from build123d import *

# Parameters (mm, degrees)
ESBO_O1_R                     = 1.5
RESSALTO_EXTRUS_O1_DEPTH      = 9
RESSALTO_EXTRUS_O2_DEPTH      = 5
RESSALTO_EXTRUS_O2_DEPTH_BACK = 11
ESBO_O2_W                     = 11
ESBO_O2_H                     = 8
FILETE1_R                     = 2.5
CHANFRO1_SIZE                 = 2


with BuildPart() as part:
    # Esboço1 → Ressalto-extrusão1 (new body)
    with BuildSketch(Plane.XY):
        Polygon((-3, -3), (3, -3), (3, 3), (-3, 3), (-10, 3), (-10, -3), align=None)
        Circle(ESBO_O1_R, mode=Mode.SUBTRACT)
    extrude(amount=RESSALTO_EXTRUS_O1_DEPTH)

    # Esboço2 → Ressalto-extrusão2 (add, two sides: drawn at the far end of the back side and taken through both)
    with BuildSketch(Plane.XZ.offset(3).offset(-RESSALTO_EXTRUS_O2_DEPTH_BACK)):
        with Locations((-15.5, -1)):
            Rectangle(ESBO_O2_W, ESBO_O2_H)
    extrude(amount=RESSALTO_EXTRUS_O2_DEPTH + RESSALTO_EXTRUS_O2_DEPTH_BACK)

    # Filete1
    # the kernel refuses this fillet: 2.5 mm, written as the material it takes off along each edge
    with BuildSketch(Plane(origin=(-10, -3, 0), x_dir=(0, 0, 1), z_dir=(1, 0, 0))) as filete1_piece_1:
        with BuildLine():
            CenterArc((FILETE1_R, -FILETE1_R), FILETE1_R, 90, 90)
            Line((0, -FILETE1_R), (0, 0))
            Line((0, 0), (FILETE1_R, 0))
        make_face()
    extrude(amount=19.25, mode=Mode.SUBTRACT)
    with BuildSketch(Plane(origin=(9.25, 3, 0), x_dir=(0, -1, 0), z_dir=(-1, 0, 0))) as filete1_piece_2:
        with BuildLine():
            CenterArc((FILETE1_R, FILETE1_R), FILETE1_R, 180, 90)
            Line((0, FILETE1_R), (0, 0))
            Line((0, 0), (FILETE1_R, 0))
        make_face()
    extrude(amount=19.25, mode=Mode.SUBTRACT)
    # the kernel refuses this fillet: 2.5 mm, written as the material it adds along each edge
    with BuildSketch(Plane(origin=(-10, -3, 2.5), x_dir=(1, 0, 0), z_dir=(0, 0, 1)), Plane(origin=(-10, 3, 2.5), x_dir=(0, 1, 0), z_dir=(0, 0, 1))) as filete1_2_piece_1:
        with BuildLine():
            CenterArc((FILETE1_R, -FILETE1_R), FILETE1_R, 90, 90)
            Line((0, -FILETE1_R), (0, 0))
            Line((0, 0), (FILETE1_R, 0))
        make_face()
    extrude(amount=0.5)
    with BuildSketch(Plane(origin=(-10, 0.5, 0), x_dir=(0, 0, -1), z_dir=(0, -1, 0))) as filete1_2_piece_2:
        with BuildLine():
            CenterArc((FILETE1_R, FILETE1_R), FILETE1_R, 180, 90)
            Line((0, FILETE1_R), (0, 0))
            Line((0, 0), (FILETE1_R, 0))
        make_face()
    extrude(amount=1)
    with BuildSketch(Plane(origin=(-10, 0.5, 2.5), x_dir=(0, 0, -1), z_dir=(0, -1, 0))) as filete1_2_piece_3:
        with BuildLine():
            CenterArc((2.5 + FILETE1_R, FILETE1_R), FILETE1_R, 180, 90)
            Line((2.5, FILETE1_R), (2.5, 0))
            Line((2.5, 0), (2.5 + FILETE1_R, 0))
        make_face()
    revolve(axis=Axis((-10, 0.5, 2.5), (1, 0, 0)), revolution_arc=90)
    with BuildSketch(Plane(origin=(-10, -0.5, 2.5), x_dir=(0, -1, 0), z_dir=(0, 0, 1))) as filete1_2_piece_4:
        with BuildLine():
            CenterArc((2.5 + FILETE1_R, FILETE1_R), FILETE1_R, 180, 90)
            Line((2.5, FILETE1_R), (2.5, 0))
            Line((2.5, 0), (2.5 + FILETE1_R, 0))
        make_face()
    revolve(axis=Axis((-10, -0.5, 2.5), (1, 0, 0)), revolution_arc=90)

    # Chanfro1
    chanfro1_edges = [part.edges().sort_by_distance(p)[0] for p in [
        (-21, 0, -5),
        (-21, 0, 3),
    ]]
    chamfer(chanfro1_edges, length=CHANFRO1_SIZE)


solid = part.part
The model under review builds one solid part; all positions refer to its coordinate system, in mm. A direction names the side the tool comes from. Round coordinates to 2 decimals unless told otherwise and drop trailing zeros. Loops run counter-clockwise (first coordinate to the right, second up) from the corner with the lowest first, then second, coordinate; pieces in that order, holes last. Notation, with made-up numbers: M -32.75,32 L -15.75,32 A10 cw -15.75,47 Z; hole C 11.5,63 d8. An arc over 180 degrees is marked long. Answer as CSV lines item,"result". Start each with the question number.
Item 1: For faces 1 (the face through (-4, 0, 9)), 2 (the face through (-2.177, 2.287, 0.752)), 3 (the face through (-10, 0, -3)), 4 (the face through (-2.324, -2.287, 0.752)), 5 (the face through (2, 0, 0)), list the 3-axis set-ups (+Z, -Z, +X, -X, +Y, -Y) from which the entire face can be reached by the end or side of a thin tool; tool diameter is ignored.
Item 2: Consider section A-A (y = 0). Write out the cut boundary in (x, z), then the cut area to 3 significant figures.
Item 3: Consider section B-B (x = 0). Write out the cut boundary in (y, z).
Item 4: Insertion check: P1, Ø3, axis at x = -4.5, z = 4.5, coming from the -Y side; P2, Ø5, axis at x = -6, z = 5, coming from the +Y side; P3, Ø1, axis at x = -6, z = 0.5, coming from the -Y side. Each pin has a flat end and moves straight along its axis. Give the tip position at first contact, or say it passes through.
Item 5: Wall thickness on line 1 (X direction, y = 0, z = 6); line 2 (Y direction, x = 0, z = 3); line 3 (X direction, y = 0.5, z = 6): over which ranges is each line inside the solid? List them lowest first. Write a range as [from, to].
Item 6: Consider section C-C (x = -6). Write out the cut boundary in (y, z), then the cut area to 3 significant figures.
Item 7: Mouldability with a two-part tool opening along Y and no side actions: class faces 6 (the face through (-1.5, 0.07, 4.44)), 7 (the face through (-4, 0, 0)), 8 (the face through (-9.248, -3.713, 2.746)) as released by +Y, released by -Y, zero draft, split by the parting line, or undercut.
Item 8: Consider section D-D (y = 6). Write out the cut boundary in (x, z).
Answer:
1,face 1,"+Z, +X, -X, +Y, -Y"
1,face 2,"-Z, +X, +Y"
1,face 3,"-Z, +X"
1,face 4,"-Z, +X, -Y"
1,face 5,"-Z, +X, +Y, -Y"
2,outline,"M -21,-3 L -19,-5 L -10,-5 L -10,-2.5 A2.5 cw -7.5,0 L -1.5,0 L -1.5,9 L -10,9 L -10,3 L -19,3 L -21,1 Z; M 1.5,0 L 3,0 L 3,9 L 1.5,9 Z"
2,area,"175 mm^2"
3,outline,"M -3,2.5 A2.5 ccw -1.5,0.21 L -1.5,9 L -3,9 Z; M 1.5,0.21 A2.5 ccw 3,2.5 L 3,9 L 1.5,9 Z"
4,P1,"stops at y = -3"
4,P2,"stops at y = 3"
4,P3,"stops at y = -2.5"
5,line 1,"x = [-10, -1.5], [1.5, 3]"
5,line 2,"y = [-3, -1.5], [1.5, 3]"
5,line 3,"x = [-10, -1.41], [1.41, 3]"
6,outline,"M -3,2.5 A2.5 ccw -0.5,0 L 0.5,0 A2.5 ccw 3,2.5 L 3,9 L -3,9 Z"
6,area,"51.3 mm^2"
7,face 6,"undercut"
7,face 7,"zero draft"
7,face 8,"released by -Y"
8,outline,"M -21,-3 L -19,-5 L -10,-5 L -10,3 L -19,3 L -21,1 Z"
